Autodesk Inventor part; units mm, degrees
ref_plane "YZ Plane" through (0, 0, 0) normal (1, 0, 0) x (0, 1, 0)
ref_plane "XZ Plane" through (0, 0, 0) normal (0, 1, 0) x (-1, 0, 0)
ref_plane "XY Plane" through (0, 0, 0) normal (0, 0, 1) x (1, 0, 0)
sketch "Sketch1" plane through (0, 0, 0) normal (0, 0, 1) x (1, 0, 0)
  line L0 (0, 0) -> (-10.5, 0)
  line L1 (-10.5, 0) -> (-10.5, -3)
  line L2 (-10.5, -3) -> (-4.5, -3)
  line L3 (-4.5, -3) -> (-4.5, -2.5)
  line L4 (-4.5, -2.5) -> (-3, -2.5)
  line L5 (-3, -2.5) -> (-3, -10)
  line L6 (-3, -10) -> (0, -10)
  line L7 (0, -10) -> (0, -1.6547)
  line L8 (0, -1.6547) -> (2, -0.5)
  line L9 (2, -0.5) -> (2, 0)
  line L10 (2, 0) -> (0, 0)
  dimension "d0" = 0.5
  dimension "d3" = 3
  dimension "d5" = 2.5
  dimension "d6" = 10
  dimension "d7" = 10.5
  dimension "d8" = 2
  dimension "d9" = 30
  dimension "d10" = 7.5
  dimension "d11" = 6
revolve "Revolution1" add sketch "Sketch1" angle 360 about axis through (0, 0, 0) along (-1, 0, 0)
sketch "Sketch2" plane through (0, 0, 0) normal (1, 0, 0) x (0, 0, -1)
  circle A0 centre (0, 0) radius 10
  circle A1 centre (0, 0) radius 1.6547
  line L0 (0, 4.0415) -> (3.5, 2.0207)
  line L1 (3.5, 2.0207) -> (3.5, -2.0207)
  line L2 (3.5, -2.0207) -> (0, -4.0415)
  line L3 (0, -4.0415) -> (-3.5, -2.0207)
  line L4 (-3.5, -2.0207) -> (-3.5, 2.0207)
  line L5 (-3.5, 2.0207) -> (0, 4.0415)
  dimension "d13" = 7
extrude "Extrusion1" cut sketch "Sketch2" against normal up to surface (3 mm away) contours A0
properties part number "nozzle"
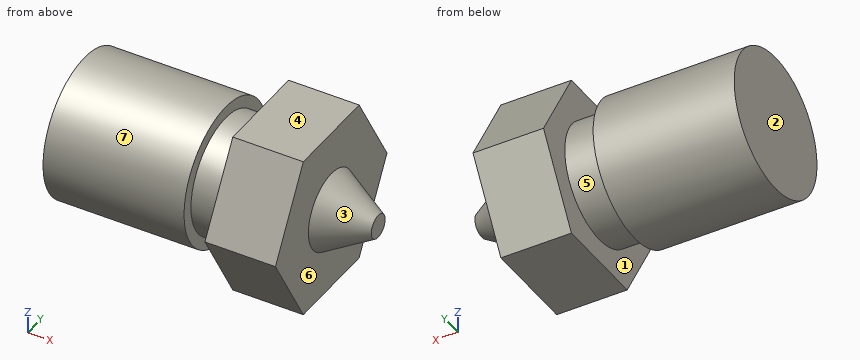
Read the model definition and answer for the solid it produces. Units are mm, in the model's axes. Face numbers are marked on the shaded views. A direction names the side the tool comes from. Round coordinates to 2 decimals unless told otherwise and drop trailing zeros. Loops run counter-clockwise (first coordinate to the right, second up) from the corner with the lowest first, then second, coordinate; pieces in that order, holes last. Notation, with made-up numbers: (23.5, -36) - (37.5, -36) arc R28 cw to (37.5, -16) - close; hole circle Ø8 at (55.5, 36). An arc over 180 degrees is marked (long way). One line per question, with ' | ' between items. Start each with the question number.
Q1. A flat-ended cylindrical pin translates along its axis: pin 1 (4 mm diameter, centred on y = -2.5, z = -1.5, fed in from +X). Find the tip coordinate at first contact, or state that the pin passes through.
Q2. Section C-C on y = 2.25 is taken. Give the vertices of the cut face in (x, z).
Q3. Section B-B on x = -5 is taken. Give the vertices of the cut face in (y, z), plus the area to 3 significant figures.
Q4. For a pull along X with two mould halves and no side action, classify the marked faces 1, 2, 3 and 4 as +X half, -X half, draft (parallel to the pull), parting line (faces both ways), or undercut.
Q5. Find the intervals of material crossed by L1, parallel to X at y = -1, z = 1.75; L2, parallel to X at y = -3, z = 1; L3, parallel to Y at x = -6.25, z = -2.5, in increasing order.
Q6. For the marked faces 5, 6 and 7, determine the directions among +Z, -Z, +X, -X, +Y, -Y from which every point of the face is accessible in a straight line to the end or side of a thin tool.
Q7. Section A-A on y = 0 is taken. Give the vertices of the cut face in (x, z), plus the area to 3 significant figures.
Established:
1) pin 1: x = 1.28
2) outline: (-10.5, -1.98) - (-4.5, -1.98) - (-4.5, -1.09) - (-3, -1.09) - (-3, -3.1) - (0, -3.1) - (0, 3.1) - (-3, 3.1) - (-3, 1.09) - (-4.5, 1.09) - (-4.5, 1.98) - (-10.5, 1.98) - close
3) outline: circle Ø6 at (0, 0) | area: 28.3 mm²
4) face 1: undercut | face 2: -X half | face 3: +X half | face 4: draft
5) L1: -10.5 to 0 | L2: -3 to 0 | L3: -1.66 to 1.66
6) face 5: none | face 6: +X | face 7: -X
7) outline: (-10.5, -3) - (-4.5, -3) - (-4.5, -2.5) - (-3, -2.5) - (-3, -3.5) - (0, -3.5) - (0, -1.65) - (2, -0.5) - (2, 0.5) - (0, 1.65) - (0, 3.5) - (-3, 3.5) - (-3, 2.5) - (-4.5, 2.5) - (-4.5, 3) - (-10.5, 3) - close | area: 68.8 mm²
